Can you work these out from the model? Positions are in its coordinate system, mm. A direction names the side the tool comes from. Coordinates: 2 decimals unless noted, no trailing zeros. Order: outer loops, then holes, each group sorted by start corner. A loop starts at its lowest first (then second) coordinate and runs counter-clockwise, first axis right, second up. Notation, with made-up numbers: M 24,-4 L 72,-4 A33 cw 72,30 Z; hole C -15.5,58 d3. An arc over 180 degrees is marked long. Answer as a JSON object with one key per item and string values.
from build123d import *

# Parameters (mm, degrees)
SKETCH1_W                      = 22.1
SKETCH1_H                      = 5.1
SKETCH2_R                      = 14.75
BOSS_EXTRUDE1_DEPTH            = 34.9
SKETCH3_R                      = 11.7
BOSS_EXTRUDE2_DEPTH            = 19.1
SKETCH4_R                      = 7.8
BOSS_EXTRUDE3_DEPTH            = 9.9
M10_CLEARANCE_HOLE1_D          = 12.7
M10_CLEARANCE_HOLE1_DEPTH      = 18.81
M10_CLEARANCE_HOLE1_TIP        = 3.815464931
F_2_2_2_2_DIAMETER_HOLE1_D     = 2.2
F_2_2_2_2_DIAMETER_HOLE1_DEPTH = 15
M3_CLEARANCE_HOLE1_D           = 3.53
M3_CLEARANCE_HOLE1_DEPTH       = 69
CHAMFER1_SIZE                  = 2


with BuildPart() as part:
    # Sketch1 → Revolve1 (revolve)
    with BuildSketch(Plane.XZ, mode=Mode.PRIVATE) as revolve1_sk:
        with Locations((11.05, 2.55)):
            Rectangle(SKETCH1_W, SKETCH1_H)
    revolve(revolve1_sk.sketch.rotate(Axis((0, 0, 5.1), (0, 0, -1)), 180), axis=Axis((0, 0, 5.1), (0, 0, -1)))

    # Sketch2 → Boss-Extrude1 (add)
    with BuildSketch(Plane.XY.offset(5.1)):
        Circle(SKETCH2_R)
    extrude(amount=BOSS_EXTRUDE1_DEPTH)

    # Sketch3 → Boss-Extrude2 (add)
    with BuildSketch(Plane.XY.offset(40)):
        Circle(SKETCH3_R)
    extrude(amount=BOSS_EXTRUDE2_DEPTH)

    # Sketch4 → Boss-Extrude3 (add)
    with BuildSketch(Plane.XY.offset(59.1)):
        Circle(SKETCH4_R)
    extrude(amount=BOSS_EXTRUDE3_DEPTH)

    # M10 Clearance Hole1
    with Locations(Plane(origin=(0, 0, 0), x_dir=(-1, 0, 0), z_dir=(0, 0, -1))):
        with Locations((0, 0)):
            Hole(M10_CLEARANCE_HOLE1_D / 2, depth=M10_CLEARANCE_HOLE1_DEPTH)
            with Locations((0, 0, -(M10_CLEARANCE_HOLE1_DEPTH + M10_CLEARANCE_HOLE1_TIP / 2))):  # 118° drill point
                Cone(0, M10_CLEARANCE_HOLE1_D / 2, M10_CLEARANCE_HOLE1_TIP, mode=Mode.SUBTRACT)

    # Ø2.2 (2.2) Diameter Hole1
    with Locations(Plane.XY.offset(69)):
        with Locations((-3, 0), (3, 0)):
            Hole(F_2_2_2_2_DIAMETER_HOLE1_D / 2, depth=F_2_2_2_2_DIAMETER_HOLE1_DEPTH)

    # M3 Clearance Hole1
    with Locations(Plane(origin=(0, 0, 0), x_dir=(-1, 0, 0), z_dir=(0, 0, -1))):
        with Locations((0, 19.0875), (-19.0875, 0), (0, -19.0875), (19.0875, 0)):
            Hole(M3_CLEARANCE_HOLE1_D / 2, depth=M3_CLEARANCE_HOLE1_DEPTH)

    # Chamfer1
    chamfer1_edges = [part.edges().sort_by_distance(p)[0] for p in [
        (-6.35, 0, 0),
    ]]
    chamfer(chamfer1_edges, length=CHAMFER1_SIZE)


solid = part.part
Item 1: Please list where these lines run through material, in increasing order: line 1 (Y direction, x = 0, z = 2.8); line 2 (Y direction, x = 0, z = 1.35); line 3 (Z direction, x = -18, y = -11.5).
Answers follow:
{"line 1": "y = -22.1 to -20.85, -17.32 to -6.35, 6.35 to 17.32, 20.85 to 22.1", "line 2": "y = -22.1 to -20.85, -17.32 to -7, 7 to 17.32, 20.85 to 22.1", "line 3": "z = 0 to 5.1"}
Item 2: I want a section at A-A, the plane x = -18.5. Write out the boundary of the cut face in (y, z), plus the area to 3 significant figures.
Answers follow:
{"outline": "M -12.09,0 L -1.66,0 L -1.66,5.1 L -12.09,5.1 Z; M 1.66,0 L 12.09,0 L 12.09,5.1 L 1.66,5.1 Z", "area": "106 mm^2"}
Item 3: Which directions (+Z, -Z, +X, -X, +Y, -Y) give clear straight access to the entire face, cutting with the end or side of a thin tool? Please do faces 5 (the cylindrical face through (-1.38, -6.2, 10.52)), 6 (the flat face through (0, -10, 0)), 7 (the flat face through (4.6, -14.4, 5.1)).
Answers follow:
{"face 5": "-Z", "face 6": "-Z, +X, -X, +Y, -Y", "face 7": "+Z"}
Item 4: If we mould it in two halves opening along Y, with no side actions, what happens to faces 1 (the flat face through (-9, 8, 40)), 2 (the cylindrical face through (14.07, 4.43, 22.31)), 3 (the cylindrical face through (1.95, 0.33, 61.4)), 4 (the flat face through (-3, 0, 54))? For each: pulls with the +Y half, pulls with the -Y half, needs draft (parallel to the pull), parting line crosses it, or undercut.
Answers follow:
{"face 1": "needs draft", "face 2": "parting line crosses it", "face 3": "undercut", "face 4": "undercut"}
Item 5: I want a section at C-C, the plane y = -12.5. Write out the boundary of the cut face in (x, z), plus the area to 3 significant figures.
Answers follow:
{"outline": "M -18.23,0 L 18.23,0 L 18.23,5.1 L 7.83,5.1 L 7.83,40 L -7.83,40 L -7.83,5.1 L -18.23,5.1 Z", "area": "732 mm^2"}
Item 6: I'm going to push flat-ended pins straight in: pin 1 (1.3 mm diameter, centred on x = -3, y = 0, fed in from +Z); pin 2 (4 mm diameter, centred on x = -4, z = 57.5, fed in from -Y); pin 3 (6 mm diameter, centred on x = -7.5, z = 54.5, fed in from -Y). Where does each tip first touch, or does it pass through?
Answers follow:
{"pin 1": "stops at z = 54", "pin 2": "stops at y = -11.53", "pin 3": "stops at y = -10.8"}
Item 7: I want a section at B-B, the plane z = 58. Write out the boundary of the cut face in (x, y).
Answers follow:
{"outline": "C 0,0 d23.4; hole C -3,0 d2.2; hole C 3,0 d2.2"}
Item 8: I want a section at D-D, the plane x = 10. Write out the boundary of the cut face in (y, z).
Answers follow:
{"outline": "M -19.71,0 L 19.71,0 L 19.71,5.1 L 10.84,5.1 L 10.84,40 L 6.07,40 L 6.07,59.1 L -6.07,59.1 L -6.07,40 L -10.84,40 L -10.84,5.1 L -19.71,5.1 Z"}
